Study the drawing (mm; zero at the part's minimum x, y, z) and answer. A direction names the side the tool comes from. Give positions to 0.01 mm unless a question says otherwise; leave off trailing zeros. Write each loop counter-clockwise with the first axis right and the second up, starting at its lowest first coordinate (ties: lowest second). Pieces come first, ordered by that corner, then holes. Notation, with made-up numbers: (18, 11.25) - (44, 11.25) arc R9 cw to (44, 15.25) - close; hole circle Ø11 at (48.25, -9.75). An arc over 180 degrees is marked (long way). Write each question's results on one line, items separated by ' | '. Start each with the question number.
Q1. Section A-A (y = 7.5) is taken. Determine the outline of the cut face in (x, z) (1 decimal).
Q2. Section C-C (z = 73) is taken. Determine the outline of the cut face in (x, y) (1 decimal).
Q3. For a pull along X with two mould halves and no side action, classify the marked faces 1, 2 and 3 as pulls with the +X half, pulls with the -X half, needs draft (parallel to the pull), parting line crosses it, or undercut.
Q4. Find the intervals of material crossed by probe 1 along X at (y, z) = (13, 8) (1 decimal); probe 2 along Y at (x, z) = (35.5, 11) (1 decimal), in increasing order.
Q5. For the marked faces 4 and 5, determine the directions among +Z, -Z, +X, -X, +Y, -Y from which every point of the face is accessible in a straight line to the end or side of a thin tool.
Q6. Section B-B (x = 40.5) is taken. Determine the outline of the cut face in (y, z) (1 decimal).
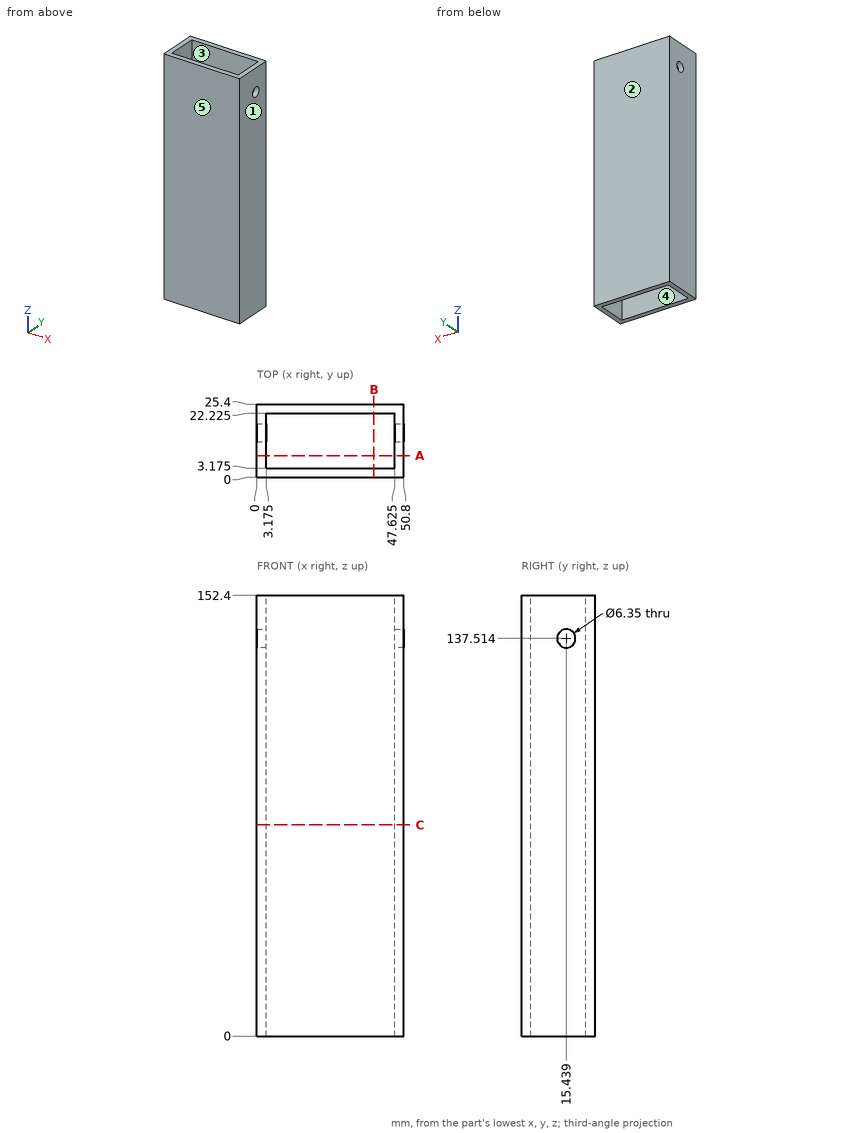
Answers below:
1) outline: (0, 0) - (3.2, 0) - (3.2, 152.4) - (0, 152.4) - close; (47.6, 0) - (50.8, 0) - (50.8, 152.4) - (47.6, 152.4) - close
2) outline: (0, 0) - (50.8, 0) - (50.8, 25.4) - (0, 25.4) - close; hole (3.2, 3.2) - (47.6, 3.2) - (47.6, 22.2) - (3.2, 22.2) - close
3) face 1: pulls with the +X half | face 2: needs draft | face 3: undercut
4) probe 1: x = 0 to 3.2, 47.6 to 50.8 | probe 2: y = 0 to 3.2, 22.2 to 25.4
5) face 4: +Z, -Z | face 5: +Z, -Z, +X, -X, -Y
6) outline: (0, 0) - (3.2, 0) - (3.2, 152.4) - (0, 152.4) - close; (22.2, 0) - (25.4, 0) - (25.4, 152.4) - (22.2, 152.4) - close
